Read the model definition and answer for the solid it produces. Units are mm, in the model's axes. A direction names the side the tool comes from. Coordinates: 2 decimals unless noted, no trailing zeros. Loops run counter-clockwise (first coordinate to the right, second up) from the corner with the lowest first, then second, coordinate; pieces in that order, holes last. Notation, with made-up numbers: (88, 10.25) -> (111, 10.25) arc R19 ccw to (111, 25.25) -> close; hole circle Ø2 at (44.5, 9). An arc over 180 degrees is marked (long way). Answer in a Markdown table with one row per item.
```python
from build123d import *

# Parameters (mm, degrees)
SKETCH1_W                                     = 74.5
SKETCH1_H                                     = 60.5
SKETCH1_R                                     = 7.1
CONSERVATIVE_MANUFACTURER_CASE_ENVELOPE_DEPTH = 108.9
D50_PILOT_ENVELOPE_START                      = -2
SKETCH2_R                                     = 25
SKETCH2_R_2                                   = 7.1
D50_PILOT_ENVELOPE_DEPTH                      = 2


with BuildPart() as part:
    # Sketch1 → Conservative_Manufacturer_Case_Envelope (new body)
    with BuildSketch(Plane.XY):
        Rectangle(SKETCH1_W, SKETCH1_H)
        Circle(SKETCH1_R, mode=Mode.SUBTRACT)
    extrude(amount=CONSERVATIVE_MANUFACTURER_CASE_ENVELOPE_DEPTH)

    # Sketch2 → D50_Pilot_Envelope (add)
    with BuildSketch(Plane.XY.offset(D50_PILOT_ENVELOPE_START)):
        Circle(SKETCH2_R)
        Circle(SKETCH2_R_2, mode=Mode.SUBTRACT)
    extrude(amount=D50_PILOT_ENVELOPE_DEPTH)


solid = part.part
```
1. Given pin 1 Ø18 at (x, y) = (4.5, 5) entering from -Z; pin 2 Ø1.5 at (x, y) = (23.5, 11) entering from -Z, each flat-ended and moving along its own axis, determine where each tip first touches the part or whether it passes through.
A:
| item | result |
|---|---|
| pin 1 | stops at z = -2 |
| pin 2 | stops at z = 0 |
2. A cutting plane is placed at B-B on y = 0. Give the vertices of the cut face in (x, z), and give its area (3 significant figures).
A:
| item | result |
|---|---|
| outline | (-37.25, 0) -> (-25, 0) -> (-25, -2) -> (-7.1, -2) -> (-7.1, 108.9) -> (-37.25, 108.9) -> close; (7.1, -2) -> (25, -2) -> (25, 0) -> (37.25, 0) -> (37.25, 108.9) -> (7.1, 108.9) -> close |
| area | 6,640 mm2 |
3. Find the intervals of material crossed by probe 1 along Y at (x, z) = (0, 73); probe 2 along Z at (x, y) = (-30, -13); probe 3 along Y at (x, z) = (-5.5, 32.5), in increasing order.
A:
| item | result |
|---|---|
| probe 1 | y = -30.25 to -7.1, 7.1 to 30.25 |
| probe 2 | z = 0 to 108.9 |
| probe 3 | y = -30.25 to -4.49, 4.49 to 30.25 |
4. A tool of negligible diameter and unlimited length cuts with its end or side. For faces 5 (the flat face through (-1, -30.25, 54)), 6 (the flat face through (-25.4, 0.4, 0)), from which of +Z, -Z, +X, -X, +Y, -Y can it reach the whole face along a straight path? Write none if from no direction.
A:
| item | result |
|---|---|
| face 5 | +Z, -Z, +X, -X, -Y |
| face 6 | -Z |
5. A cutting plane is placed at C-C on z = 29.5. Give the vertices of the cut face in (x, y), and give its area (3 significant figures).
A:
| item | result |
|---|---|
| outline | (-37.25, -30.25) -> (37.25, -30.25) -> (37.25, 30.25) -> (-37.25, 30.25) -> close; hole circle Ø14.2 at (0, 0) |
| area | 4,350 mm2 |
6. A cutting plane is placed at A-A on x = 0. Give the vertices of the cut face in (y, z), and give its area (3 significant figures).
A:
| item | result |
|---|---|
| outline | (-30.25, 0) -> (-25, 0) -> (-25, -2) -> (-7.1, -2) -> (-7.1, 108.9) -> (-30.25, 108.9) -> close; (7.1, -2) -> (25, -2) -> (25, 0) -> (30.25, 0) -> (30.25, 108.9) -> (7.1, 108.9) -> close |
| area | 5,110 mm2 |
7. The mould has two halves that part along X. Classify faces 1 (the flat face through (-1, 30.25, 54)), 2 (the flat face through (37.25, 0, 54)), 3 (the cylindrical face through (-0.92, 7.04, 52.67)), 4 (the cylindrical face through (23.846, 7.509, -1.014)): pulls with the +X half, pulls with the -X half, needs draft (parallel to the pull), parting line crosses it, or undercut.
A:
| item | result |
|---|---|
| face 1 | needs draft |
| face 2 | pulls with the +X half |
| face 3 | undercut |
| face 4 | parting line crosses it |
